```python
from build123d import *

# Parameters (mm, degrees)
SKETCH1_W           = 317.5
SKETCH1_H           = 101.6
BOSS_EXTRUDE1_DEPTH = 8.0518
BOSS_EXTRUDE2_START = 8.0518
SKETCH2_W           = 317.5
SKETCH2_H           = 8.128
BOSS_EXTRUDE2_DEPTH = 103.378
BOSS_EXTRUDE3_START = 8.0518
SKETCH3_W           = 9.525
SKETCH3_H           = 46.5328
BOSS_EXTRUDE3_DEPTH = 76.9874
BOSS_EXTRUDE4_START = 8.0518
SKETCH3_3_W         = 9.525
SKETCH3_3_H         = 46.5328
BOSS_EXTRUDE4_DEPTH = 76.1746


with BuildPart() as part:
    # Sketch1 → Boss-Extrude1 (new body)
    with BuildSketch(Plane(origin=(0, 0, 0), x_dir=(1, 0, 0), z_dir=(0, 1, 0))):
        with Locations((158.75, 50.8)):
            Rectangle(SKETCH1_W, SKETCH1_H)
    extrude(amount=BOSS_EXTRUDE1_DEPTH)

    # Sketch2 → Boss-Extrude2 (add)
    with BuildSketch(Plane(origin=(0, 0, 0), x_dir=(1, 0, 0), z_dir=(0, 1, 0)).offset(BOSS_EXTRUDE2_START)):
        with Locations((158.75, 50.5968)):
            Rectangle(SKETCH2_W, SKETCH2_H)
    extrude(amount=BOSS_EXTRUDE2_DEPTH)

    # Sketch3 → Boss-Extrude3 (add)
    with BuildSketch(Plane(origin=(0, 0, 0), x_dir=(1, 0, 0), z_dir=(0, 1, 0)).offset(BOSS_EXTRUDE3_START)):
        with Locations((6.6675, 23.2664)):
            Rectangle(SKETCH3_W, SKETCH3_H)
    extrude(amount=BOSS_EXTRUDE3_DEPTH)

    # Sketch3<3> → Boss-Extrude4 (add)
    with BuildSketch(Plane(origin=(0, 0, 0), x_dir=(1, 0, 0), z_dir=(0, 1, 0)).offset(BOSS_EXTRUDE4_START)):
        with Locations((165.1635, 23.2664)):
            Rectangle(SKETCH3_3_W, SKETCH3_3_H)
    extrude(amount=BOSS_EXTRUDE4_DEPTH)


solid = part.part
```
Input: part model. Units: mm. Frame: model coordinates. A direction names the side the tool comes from. Coordinates: 2 decimals unless noted, no trailing zeros. Write each loop counter-clockwise with the first axis right and the second up, starting at its lowest first coordinate (ties: lowest second). Pieces come first, ordered by that corner, then holes.
1) Pin query (flat end, axial travel): pin 1 Ø14 at (y, z) = (36, -13) entering from +X; pin 2 Ø4 at (x, y) = (219, 18) entering from -Z; pin 3 Ø10.5 at (x, z) = (5, -26.5) entering from +Y. Return the tip coordinate at first contact, or that it passes through.
2) Section D-D on z = -93. Output: boundary loops of the cut face in (x, y), and give its area (3 significant figures).
3) Mould query, pull axis X, two halves, no side actions, for faces 4 (the flat face through (243, 8.052, -24)), 5 (the flat face through (11.43, 46, -23)), 6 (the flat face through (1.905, 46, -23)). Classes: pulls with the +X half, pulls with the -X half, needs draft (parallel to the pull), parting line crosses it, or undercut.
4) Material intervals for line 1 along X through (y, z) = (35, -9.5) (3 decimals); line 2 along Y through (x, z) = (82, -36.5); line 3 along Z through (x, y) = (31, 94), sorted ascending.
5) Section C-C on x = 232.5. Output: boundary loops of the cut face in (y, z).
6) Section B-B on y = 54. Output: boundary loops of the cut face in (x, z) (3 decimals), and give its area (3 significant figures).
7) Set-up query: faces 1 (the flat face through (160.401, 46, -23)), 2 (the flat face through (157, 8.052, -78)), 3 (the flat face through (169.926, 46, -23)). Return all of +Z, -Z, +X, -X, +Y, -Y with unobstructed straight access to the full face (end or side cutting, diameter ignored); none if empty.
8) Section A-A on z = -10.5. Output: boundary loops of the cut face in (x, y) (3 decimals), and give its area (3 significant figures).
Check result:
1. pin 1: stops at x = 169.93
1. pin 2: stops at z = -54.66
1. pin 3: stops at y = 85.04
2. outline: (0, 0) - (317.5, 0) - (317.5, 8.05) - (0, 8.05) - close
2. area: 2,560 mm2
3. face 4: needs draft
3. face 5: undercut
3. face 6: pulls with the -X half
4. line 1: x = 1.905 to 11.43, 160.401 to 169.926
4. line 2: y = 0 to 8.05
4. line 3: z = -54.66 to -46.53
5. outline: (0, -101.6) - (8.05, -101.6) - (8.05, -54.66) - (111.43, -54.66) - (111.43, -46.53) - (8.05, -46.53) - (8.05, 0) - (0, 0) - close
6. outline: (0, -54.661) - (317.5, -54.661) - (317.5, -46.533) - (169.926, -46.533) - (169.926, 0) - (160.401, 0) - (160.401, -46.533) - (11.43, -46.533) - (11.43, 0) - (1.905, 0) - (1.905, -46.533) - (0, -46.533) - close
6. area: 3,470 mm2
7. face 1: +Z, +Y
7. face 2: -Z, +X, -X, +Y
7. face 3: +Z, +X, +Y
8. outline: (0, 0) - (317.5, 0) - (317.5, 8.052) - (169.926, 8.052) - (169.926, 84.226) - (160.401, 84.226) - (160.401, 8.052) - (11.43, 8.052) - (11.43, 85.039) - (1.905, 85.039) - (1.905, 8.052) - (0, 8.052) - close
8. area: 4,020 mm2
